Design review of the part built by this model. Coordinates are the model's own, in mm. A direction names the side the tool comes from. Give positions to 0.01 mm unless a question says otherwise; leave off trailing zeros. Order: outer loops, then holes, each group sorted by start corner. A loop starts at its lowest first (then second) coordinate and runs counter-clockwise, first axis right, second up. Notation, with made-up numbers: (-13, 87.25) -> (-8, 87.25) arc R26 cw to (-8, 106.25) -> close; hole circle Ø2 at (16, 71.5). An arc over 180 degrees is marked (long way). One line per item, written item: value.
Autodesk Inventor part; units mm, degrees
ref_plane "YZ Plane" through (0, 0, 0) normal (1, 0, 0) x (0, 1, 0)
ref_plane "XZ Plane" through (0, 0, 0) normal (0, 1, 0) x (-1, 0, 0)
ref_plane "XY Plane" through (0, 0, 0) normal (0, 0, 1) x (1, 0, 0)
sketch "Sketch1" plane through (0, 0, 0) normal (0, 0, 1) x (1, 0, 0)
  line L0 (0, -36.3851) -> (0, 36.5144) construction
  circle A0 centre (0, 0.0647) radius 20
  circle A1 centre (0, 20.0647) radius 4.05
  circle A2 centre (0, -19.9353) radius 4.05
  line L1 (7.5, -24.9353) -> (-7.5, -24.9353)
  line L2 (-12.5, -19.9353) -> (-12.5, 20.0647)
  line L3 (-7.5, 25.0647) -> (7.5, 25.0647)
  line L4 (12.5, 20.0647) -> (12.5, -19.9353)
  line L5 (12.5, -24.9353) -> (-12.5, 25.0647) construction
  line L6 (-12.5, -24.9353) -> (12.5, 25.0647) construction
  arc A3 (-7.5, 25.0647) -> (-12.5, 20.0647) centre (-7.5, 20.0647) ccw
  arc A4 (12.5, 20.0647) -> (7.5, 25.0647) centre (7.5, 20.0647) ccw
  arc A5 (7.5, -24.9353) -> (12.5, -19.9353) centre (7.5, -19.9353) ccw
  arc A6 (-12.5, -19.9353) -> (-7.5, -24.9353) centre (-7.5, -19.9353) ccw
  circle A7 centre (0, 0.0647) radius 7.5
  dimension "d6" = 40
  dimension "d7" = 8.1
  dimension "d8" = 8.1
  dimension "d9" = 25
  dimension "d10" = 50
  dimension "d11" = 5
  dimension "d12" = 15
extrude "Extrusion1" add sketch "Sketch1" along normal blind 3 contours L4 A0 A2 L2 A1 | A0 A1 L2 A3 L3 A4 L4 | L4 A5 L1 A6 L2 A0 A2
sketch "Skizze2" plane through (0, 0, 3) normal (0, 0, 1) x (1, 0, 0)
  circle A0 centre (0, 20.0647) radius 4.05
  circle A1 centre (0, 0.0647) radius 7.5
  circle A2 centre (0, -19.9353) radius 4.05
  arc A3 (12.5, 20.0647) -> (7.5, 25.0647) centre (7.5, 20.0647) ccw
  line L0 (7.5, 25.0647) -> (-7.5, 25.0647)
  arc A4 (-7.5, 25.0647) -> (-12.5, 20.0647) centre (-7.5, 20.0647) ccw
  line L1 (-12.5, 20.0647) -> (-12.5, -19.9353)
  arc A5 (-12.5, -19.9353) -> (-7.5, -24.9353) centre (-7.5, -19.9353) ccw
  line L2 (-7.5, -24.9353) -> (7.5, -24.9353)
  arc A6 (7.5, -24.9353) -> (12.5, -19.9353) centre (7.5, -19.9353) ccw
  line L3 (12.5, -19.9353) -> (12.5, 20.0647)
  point P0 (0, 0)
extrude "Extrusion2" add sketch "Skizze2" along normal blind 0.6 contours A0 | A2 | L3 A6 L2 A5 L1 A4 L0 A3
properties part number "20_Cube_Insert_Sample_clamp"
Item 1: Draft analysis for pull direction Y (two halves, no side actions). For faces 1 (the cylindrical face through (-10.996, -23.509, 1.775)), 2 (the cylindrical face through (-0.53, -23.95, 1.48)), 3 (the flat face through (12.5, 0, 2)), state which applies: pulls with the +Y half, pulls with the -Y half, needs draft (parallel to the pull), parting line crosses it, or undercut.
Returned:
face 1: pulls with the -Y half
face 2: undercut
face 3: needs draft
Item 2: Machinability: for faces 4 (the flat face through (0, -20, 3)), 5 (the cylindrical face through (10.996, 23.639, 1.775)), which of the approach directions +Z, -Z, +X, -X, +Y, -Y give a long, thin tool a straight path to every point of the face, cutting with its end or side? Answer none if there is none.
Returned:
face 4: -Z
face 5: +Z, -Z, +X, +Y
Item 3: Add section A-A on x = 0. Give the boundary of the cut face in (y, z), plus the area to 3 significant figures.
Returned:
outline: (-24.94, 0) -> (-23.99, 0) -> (-23.99, 3) -> (-15.89, 3) -> (-15.89, 0) -> (-7.44, 0) -> (-7.44, 3.6) -> (-24.94, 3.6) -> close; (7.56, 0) -> (16.01, 0) -> (16.01, 3) -> (24.11, 3) -> (24.11, 0) -> (25.06, 0) -> (25.06, 3.6) -> (7.56, 3.6) -> close
area: 77.4 mm²
Item 4: To check wall thickness, follow line 1 along Y through (x, z) = (0, 1); line 2 along X through (y, z) = (20, 2.2); line 3 along X through (y, z) = (18, 1.15). State the ranges of each line that lie inside material, in increasing order. Write a range as from..to.
Returned:
line 1: -24.94..-23.99, -15.89..-7.44, 7.56..16.01, 24.11..25.06
line 2: -12.5..-4.05, 4.05..12.5
line 3: -12.5..-3.48, 3.48..12.5
Item 5: Clearance check with flat-ended pins moving along their axes: P1, Ø2.5, axis at x = 1.5, y = -19.5, coming from the -Z side; P2, Ø12, axis at x = 0, y = 0.06, coming from the -Z side. State where each tip first meets the part, or that it passes through.
Returned:
P1: z = 3
P2: through
Item 6: Add section B-B on z = 1.65. Give the boundary of the cut face in (x, y), plus the area to 3 significant figures.
Returned:
outline: (-12.5, -19.94) arc R5 ccw to (-7.5, -24.94) -> (7.5, -24.94) arc R5 ccw to (12.5, -19.94) -> (12.5, 20.06) arc R5 ccw to (7.5, 25.06) -> (-7.5, 25.06) arc R5 ccw to (-12.5, 20.06) -> close; hole circle Ø15 at (0, 0.06); hole circle Ø8.1 at (0, -19.94); hole circle Ø8.1 at (0, 20.06)
area: 949 mm²
Item 7: Add section C-C on y = -20.5. Give the boundary of the cut face in (x, z).
Returned:
outline: (-12.47, 0) -> (-4.01, 0) -> (-4.01, 3) -> (4.01, 3) -> (4.01, 0) -> (12.47, 0) -> (12.47, 3.6) -> (-12.47, 3.6) -> close
